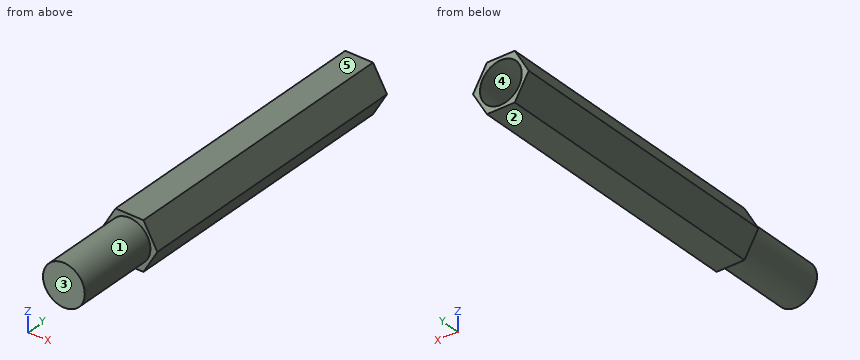
```python
from build123d import *

# Parameters (mm, degrees)
EXTRUDE_1_DEPTH           = 21
SKETCH_2_W                = 1.5
SKETCH_2_H                = 6
HOLE_WIZARD_3_0_3_1_D     = 3
HOLE_WIZARD_3_0_3_1_DEPTH = 5


with BuildPart() as part:
    # 草图1 → 凸台-拉伸1 (new body)
    with BuildSketch(Plane.XZ):
        Polygon((-1, 1.732050808), (-2, 0), (-1, -1.732050808), (1, -1.732050808), (2, 0), (1, 1.732050808), align=None)
    extrude(amount=-EXTRUDE_1_DEPTH)

    # 草图2 → 旋转1 (revolve)
    with BuildSketch(Plane.XY, mode=Mode.PRIVATE) as revolve_1_sk:
        with Locations((0.75, -3)):
            Rectangle(SKETCH_2_W, SKETCH_2_H)
    revolve(revolve_1_sk.sketch.rotate(Axis((0, 0, 0), (0, -1, 0)), 270), axis=Axis((0, 0, 0), (0, -1, 0)))

    # Ø3.0 (3) 直径孔1
    with Locations(Plane(origin=(0, 21, 0), x_dir=(1, 0, 0), z_dir=(0, 1, 0))):
        with Locations((0, 0)):
            Hole(HOLE_WIZARD_3_0_3_1_D / 2, depth=HOLE_WIZARD_3_0_3_1_DEPTH)


solid = part.part
```
Check sheet for the modelled part. Datum: model origin and axes. Units: mm. Face numbers are marked on the shaded views. A direction names the side the tool comes from. Coordinates: 2 decimals unless noted, no trailing zeros. Order: outer loops, then holes, each group sorted by start corner. A loop starts at its lowest first (then second) coordinate and runs counter-clockwise, first axis right, second up. Notation, with made-up numbers: (3, 72.5) -> (36, 72.5) arc R19 ccw to (36, 105.5) -> close; hole circle Ø1 at (49, 1). An arc over 180 degrees is marked (long way). Write item = value, one per line. Start each with the question number.
1) Cross-section at D-D (y = -4). Enter the section's corners in (x, z), then the cut area to 3 significant figures.
2) Access from +Z, -Z, +X, -X, +Y, -Y to the whole of each face (thin tool, end or side, straight path). Record for the marked faces 1 and 2.
3) Cross-section at C-C (z = -0.7). Enter the section's corners in (x, y).
4) Go/stop test with a flat-tipped pin: P1, Ø2, axis at x = 0, y = -2, coming from the +Z side. Record where the tip stops, or that it passes through.
5) Material ranges on L1, parallel to Z at x = 0, y = 17.45; L2, parallel to Y at x = 1.1, z = 0.7; L3, parallel to Y at x = -0.7, z = 1.4, recorded low to high.
6) Mould release check, pull along Z, two halves, no side actions. Record for the marked faces 3, 4 and 5: +Z half, -Z half, draft (parallel to the pull), parting line (faces both ways), or undercut.
7) Cross-section at A-A (y = 16.25). Enter the section's corners in (x, z), then the cut area to 3 significant figures.
8) Cross-section at B-B (x = 0). Enter the section's corners in (y, z).
Ans:
q1.outline = circle Ø3 at (0, 0)
q1.area = 7.07 mm²
q2.face_1 = -Y
q2.face_2 = -Z, +X, -X, +Y, -Y
q3.outline = (-1.6, 0) -> (-1.33, 0) -> (-1.33, -6) -> (1.33, -6) -> (1.33, 0) -> (1.6, 0) -> (1.6, 21) -> (1.33, 21) -> (1.33, 16) -> (-1.33, 16) -> (-1.33, 21) -> (-1.6, 21) -> close
q4.P1 = 1.5
q5.L1 = -1.73 to -1.5, 1.5 to 1.73
q5.L2 = -6 to 16
q5.L3 = 0 to 21
q6.face_3 = draft
q6.face_4 = undercut
q6.face_5 = +Z half
q7.outline = (-2, 0) -> (-1, -1.73) -> (1, -1.73) -> (2, 0) -> (1, 1.73) -> (-1, 1.73) -> close; hole circle Ø3 at (0, 0)
q7.area = 3.32 mm²
q8.outline = (-6, -1.5) -> (0, -1.5) -> (0, -1.73) -> (21, -1.73) -> (21, -1.5) -> (16, -1.5) -> (16, 1.5) -> (21, 1.5) -> (21, 1.73) -> (0, 1.73) -> (0, 1.5) -> (-6, 1.5) -> close
